```python
from build123d import *

# Parameters (mm, degrees)
F0_W     = 4
F0_H     = 5
F1_DEPTH = 3
F3_DEPTH = 2.5
F4_SIZE  = 0.5
F5_SIZE  = 0.5
F6_SIZE  = 0.5


with BuildPart() as f1:
    # F0 (on Front) → F1 (new body, symmetric)
    with BuildSketch(Plane.XZ):
        Polygon((6, 0), (10, 0), (10, 36), (0, 36), (0, 28.5), (2, 28.5), (2, 32.75), (8, 32.75), (8, 3.25), (2, 3.25), (2, 7.5), (0, 7.5), (0, 0), align=None)
        with BuildLine():
            ThreePointArc((0, 7.5), (-1.692811, 3.75), (0, 0))
            Line((0, 0), (0, 7.5))
        make_face()
        with BuildLine():
            Line((0, 28.5), (0, 36))
            ThreePointArc((0, 36), (-1.692811, 32.25), (0, 28.5))
        make_face()
        with Locations((8, -2.5)):
            Rectangle(F0_W, F0_H)
    extrude(amount=F1_DEPTH, both=True)

    # F2 (on face) → F3 (join)
    with BuildSketch(Plane.YZ.offset(10)):
        with BuildLine():
            ThreePointArc((-3, -5), (-1.837117, -12.462021), (4.5, -8.354102))
            ThreePointArc((4.5, -8.354102), (4.107919, -6.516985), (3, -5))
            Line((3, -5), (1, -5))
            ThreePointArc((1, -5), (2.806243, -6.262452), (3.5, -8.354102))
            ThreePointArc((3.5, -8.354102), (-2.09165, -11.160345), (-1, -5))
            Line((-1, -5), (-3, -5))
        make_face()
    extrude(amount=-F3_DEPTH)

    # F4
    f4_edges = [f1.edges().sort_by_distance(p)[0] for p in [
        (7.5, -1.837117, -12.462021),
    ]]
    chamfer(f4_edges, length=F4_SIZE)

    # F5
    f5_edges = [f1.edges().sort_by_distance(p)[0] for p in [
        (10, -1.837117, -12.462021),
    ]]
    chamfer(f5_edges, length=F5_SIZE)

    # F6
    f6_edges = [f1.edges().sort_by_distance(p)[0] for p in [
        (2, -3, 5.375),
        (5, -3, 3.25),
        (8, -3, 18),
        (2, -3, 30.625),
        (5, -3, 32.75),
        (2, 3, 5.375),
        (5, 3, 3.25),
        (8, 3, 18),
        (5, 3, 32.75),
        (2, 3, 30.625),
    ]]
    chamfer(f6_edges, length=F6_SIZE)


solid = f1.part
```
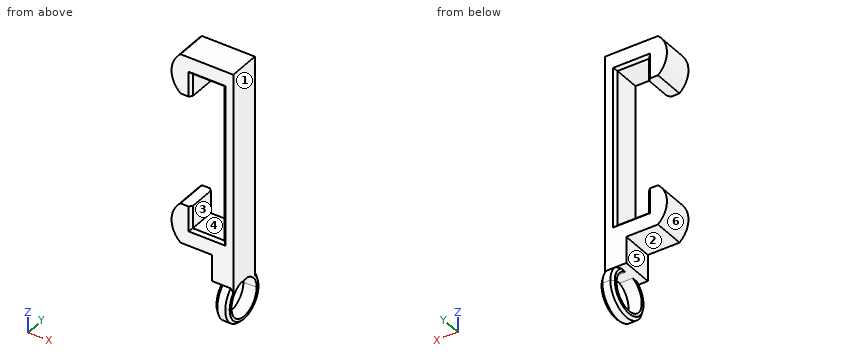
Source: CAD feature listing. Evaluate the final solid. Frame: model axes, mm. Face numbers are marked on the shaded views. A direction names the side the tool comes from. Coordinates: 2 decimals unless noted, no trailing zeros. Loops run counter-clockwise (first coordinate to the right, second up) from the corner with the lowest first, then second, coordinate; pieces in that order, holes last. Notation, with made-up numbers: M 35.25,-1.75 L 79.25,-1.75 A19 cw 79.25,30.25 Z; hole C 40,-38.5 d1. An arc over 180 degrees is marked long. Use a Markdown table: item, result. Add a question column.
Q1. Section query B-B, the plane x = 2.75. Return loops of the section in (y, z).
Q2. Draft query along X for the marked faces 1, 2 and 3. Return one class per face: pulls with the +X half, pulls with the -X half, needs draft (parallel to the pull), parting line crosses it, or undercut.
Q3. Section query A-A, the plane y = 0. Return loops of the section in (x, z), and give its area (3 significant figures).
Q4. Section query C-C, the plane z = 8. Return loops of the section in (x, y).
Q5. Section query D-D, the plane x = 0.75. Return loops of the section in (y, z).
Q6. First-contact query: pin 1 (1.2 mm diameter, centred on x = 7.5, y = -0.5, fed in from -Z); pin 2 (2.5 mm diameter, centred on y = -1, z = -1.5, fed in from -X); pin 3 (1.5 mm diameter, centred on y = 0, z = 22.5, fed in from -X); pin 4 (5 mm diameter, centred on x = 6, z = -7.5, fed in from +Y). Flat tips, straight axial feed; report the tip coordinate or a pass-through.
Q7. Material intervals for L1, parallel to Z at x = 4.75, y = 0.25; L2, parallel to Z at x = 9, y = 0; L3, parallel to X at y = 1, z = 3.5, sorted ascending.
Q8. Access query for the marked faces 4, 5 and 6. Directions: +Z, -Z, +X, -X, +Y, -Y. A direction counts if a zero-diameter tool reaches every point of the face in a straight line with its end or side. Return the directions, or none.
Result:
| question | item | result |
|---|---|---|
| 1 | outline | M -3,0 L 3,0 L 3,2.75 L 2.5,3.25 L -2.5,3.25 L -3,2.75 Z; M -3,33.25 L -2.5,32.75 L 2.5,32.75 L 3,33.25 L 3,36 L -3,36 Z |
| 2 | face 1 | pulls with the +X half |
| 2 | face 2 | needs draft |
| 2 | face 3 | undercut |
| 3 | outline | M 0,0 L 6,0 L 6,-5 L 10,-5 L 10,36 L 0,36 A5 ccw 0,28.5 L 2,28.5 L 2,32.75 L 8,32.75 L 8,3.25 L 2,3.25 L 2,7.5 L 0,7.5 A5 ccw Z; M 7.5,-12.35 L 8,-12.85 L 9.5,-12.85 L 10,-12.35 L 10,-11.85 L 7.5,-11.85 Z |
| 3 | area | 181 mm2 |
| 4 | outline | M 8,-2.5 L 8.5,-3 L 10,-3 L 10,3 L 8.5,3 L 8,2.5 Z |
| 5 | outline | M -3,0 L 3,0 L 3,7.5 L -3,7.5 Z; M -3,28.5 L 3,28.5 L 3,36 L -3,36 Z |
| 6 | pin 1 | stops at z = -12.85 |
| 6 | pin 2 | stops at x = 6 |
| 6 | pin 3 | stops at x = 8 |
| 6 | pin 4 | stops at y = 4.5 |
| 7 | L1 | z = 0 to 3.25, 32.75 to 36 |
| 7 | L2 | z = -12.85 to -11.85, -5 to 36 |
| 7 | L3 | x = -1.69 to 2, 8 to 10 |
| 8 | face 4 | +Y, -Y |
| 8 | face 5 | -Z, -X, +Y, -Y |
| 8 | face 6 | -X, +Y, -Y |
